```python
from build123d import *

# Parameters (mm, degrees)
BOSS_EXTRUDE1_DEPTH      = 30
FILLET1_R                = 10
CUT_EXTRUDE1_DEPTH       = 156.32224567
CUT_EXTRUDE1_DEPTH_BACK  = 156.32224567
SKETCH2_R                = 25
CUT_EXTRUDE2_START       = -30
SKETCH3_R                = 47.5
CUT_EXTRUDE2_DEPTH       = 10
CUT_EXTRUDE3_START       = 20
SKETCH3_3_R              = 47.5
CUT_EXTRUDE3_DEPTH       = 10
BOSS_EXTRUDE2_DEPTH      = 30
BOSS_EXTRUDE2_DEPTH_BACK = 30
SKETCH4_R                = 30
SKETCH4_R_2              = 25


with BuildPart() as part:
    # Sketch1 → Boss-Extrude1 (new, symmetric)
    with BuildSketch(Plane(origin=(0, 0, 0), x_dir=(0, 0, -1), z_dir=(1, 0, 0))):
        with BuildLine():
            Line((0, -100), (0, 100))
            Line((0, 100), (-17, 100))
            Line((-17, 100), (-17, 60))
            ThreePointArc((-17, 60), (-115, 0), (-17, -60))
            Line((-17, -60), (-17, -100))
            Line((-17, -100), (0, -100))
        make_face()
    extrude(amount=BOSS_EXTRUDE1_DEPTH, both=True)

    # Fillet1
    fillet1_edges = [part.edges().sort_by_distance(p)[0] for p in [
        (0, -60, 17),
        (0, 60, 17),
    ]]
    fillet(fillet1_edges, radius=FILLET1_R)

    # Sketch2 → Cut-Extrude1 (cut, two sides: drawn at the far end of the back side and taken through both)
    with BuildSketch(Plane(origin=(0, 0, 0), x_dir=(0, 0, -1), z_dir=(1, 0, 0)).offset(-CUT_EXTRUDE1_DEPTH_BACK)):
        with Locations((-60, 0)):
            Circle(SKETCH2_R)
    extrude(amount=CUT_EXTRUDE1_DEPTH + CUT_EXTRUDE1_DEPTH_BACK, mode=Mode.SUBTRACT)

    # Sketch3 → Cut-Extrude2 (cut)
    with BuildSketch(Plane(origin=(0, 0, 0), x_dir=(0, 0, -1), z_dir=(1, 0, 0)).offset(CUT_EXTRUDE2_START)):
        with Locations((-60, 0)):
            Circle(SKETCH3_R)
    extrude(amount=CUT_EXTRUDE2_DEPTH, mode=Mode.SUBTRACT)

    # Sketch3<3> → Cut-Extrude3 (cut)
    with BuildSketch(Plane(origin=(0, 0, 0), x_dir=(0, 0, -1), z_dir=(1, 0, 0)).offset(CUT_EXTRUDE3_START)):
        with Locations((-60, 0)):
            Circle(SKETCH3_3_R)
    extrude(amount=CUT_EXTRUDE3_DEPTH, mode=Mode.SUBTRACT)

    # Sketch4 → Boss-Extrude2 (add, two sides: drawn at the far end of the back side and taken through both)
    with BuildSketch(Plane(origin=(0, 0, 0), x_dir=(0, 0, -1), z_dir=(1, 0, 0)).offset(-BOSS_EXTRUDE2_DEPTH_BACK)):
        with Locations((-60, 0)):
            Circle(SKETCH4_R)
        with Locations((-60, 0)):
            Circle(SKETCH4_R_2, mode=Mode.SUBTRACT)
    extrude(amount=BOSS_EXTRUDE2_DEPTH + BOSS_EXTRUDE2_DEPTH_BACK)


solid = part.part
```
Here's how the part is built. I have some questions about the finished solid (model axes, mm). A direction names the side the tool comes from. Round coordinates to 2 decimals unless told otherwise and drop trailing zeros. Write each loop counter-clockwise with the first axis right and the second up, starting at its lowest first coordinate (ties: lowest second). Pieces come first, ordered by that corner, then holes. Notation, with made-up numbers: M -36.5,49.5 L -11.5,49.5 A12 cw -11.5,63.5 Z; hole C 5.25,60 d1. An arc over 180 degrees is marked long. Answer as CSV lines item,"result". Start each with the question number.
1. Thinking about a two-plate mould opening in Y: for faces 4 (the cylindrical face through (0.42, 1.736, 114.978)), 5 (the flat face through (-30, 0, 11)), 6 (the cylindrical face through (0.42, 66.53, 21.05)), 7 (the flat face through (20, -31, 61)), which applies, released by +Y, released by -Y, zero draft, split by the parting line, or undercut?
2. I need wall thicknesses on probe 1 along Y at (x, z) = (27, 63); probe 2 along Y at (x, z) = (27.5, 65); probe 3 along Z at (x, y) = (-25, 91). Which ranges of each line are inside material? Lowest first, please.
3. Suppose I cut it at B-B on z = 52. Write out the boundary of the cut face in (x, y), then the cut area to 3 significant figures.
4. Suppose I cut it at D-D on x = -6. Write out the boundary of the cut face in (y, z), then the cut area to 3 significant figures.
5. I'm going to push flat-ended pins straight in: pin 1 Ø10 at (x, z) = (1, 70.5) entering from +Y; pin 2 Ø4 at (y, z) = (-25.5, 83.5) entering from +X; pin 3 Ø5 at (x, y) = (-21.5, 77) entering from +Z. Where does each tip first touch, or does it pass through?
6. Suppose I cut it at A-A on y = 0. Write out the boundary of the cut face in (x, z), then the cut area to 3 significant figures.
7. Suppose I cut it at C-C on x = 24. Write out the boundary of the cut face in (y, z).
8. On a 3-axis mill with a long thin cutter (end or side, diameter ignored), from which of +Z, -Z, +X, -X, +Y, -Y can I reach the whole of each face in a straight line? I mean faces 1 (the flat face through (0, -87, 17)), 2 (the flat face through (-20, -31, 61)), 3 (the flat face through (0, 87, 17)). Say none if no direction works.
Check result:
1,face 4,"split by the parting line"
1,face 5,"zero draft"
1,face 6,"released by +Y"
1,face 7,"undercut"
2,probe 1,"y = -65.59 to -47.41, -29.85 to -24.82, 24.82 to 29.85, 47.41 to 65.59"
2,probe 2,"y = -65.09 to -47.24, -29.58 to -24.49, 24.49 to 29.58, 47.24 to 65.09"
2,probe 3,"z = 0 to 17"
3,outline,"M -30,-67.23 L 30,-67.23 L 30,-46.82 L 20,-46.82 L 20,-28.91 L 30,-28.91 L 30,-23.69 L -30,-23.69 L -30,-28.91 L -20,-28.91 L -20,-46.82 L -30,-46.82 Z; M -30,23.69 L 30,23.69 L 30,28.91 L 20,28.91 L 20,46.82 L 30,46.82 L 30,67.23 L -30,67.23 L -30,46.82 L -20,46.82 L -20,28.91 L -30,28.91 Z"
3,area,"4,510 mm2"
4,outline,"M -100,0 L 100,0 L 100,17 L 74.57,17 A10 cw 64.93,29.67 A67.37 ccw long -64.93,29.67 A10 cw -74.57,17 L -100,17 Z; hole C 0,60 d50"
4,area,"12,600 mm2"
5,pin 1,"stops at y = 64.95"
5,pin 2,"stops at x = 20"
5,pin 3,"stops at z = 17"
6,outline,"M -30,0 L 30,0 L 30,12.5 L 20,12.5 L 20,30 L 30,30 L 30,35 L -30,35 L -30,30 L -20,30 L -20,12.5 L -30,12.5 Z; M -30,85 L 30,85 L 30,90 L 20,90 L 20,107.5 L 30,107.5 L 30,115 L -30,115 L -30,107.5 L -20,107.5 L -20,90 L -30,90 Z"
6,area,"3,200 mm2"
7,outline,"M -100,0 L 100,0 L 100,17 L 74.57,17 A10 cw 64.93,29.67 A67.37 ccw long -64.93,29.67 A10 cw -74.57,17 L -100,17 Z; C 0,60 d60; hole C 0,60 d95; hole C 0,60 d50"
8,face 1,"+Z, +X, -X, -Y"
8,face 2,"-X"
8,face 3,"+Z, +X, -X, +Y"
